```python
from build123d import *

# Parameters (mm, degrees)
SKETCH1_R               = 20
SKETCH1_R_2             = 14.25
SKETCH1_R_3             = 1.6
SKETCH1_W               = 2
SKETCH1_H               = 20
BOSS_EXTRUDE1_DEPTH     = 2
CUT_EXTRUDE3_DEPTH      = 171.89177862
CUT_EXTRUDE3_DEPTH_BACK = 171.89177862
SKETCH4_W               = 15
SKETCH4_H               = 2
CUT_EXTRUDE4_DEPTH      = 171.89177862
CUT_EXTRUDE4_DEPTH_BACK = 171.89177862
SKETCH5_R               = 14.25
SKETCH5_R_2             = 1.6


with BuildPart() as part:
    # Sketch1 → Boss-Extrude1 (new body)
    with BuildSketch(Plane.XY):
        Polygon((-158, -56), (-146.5, -56), (-146.5, -60), (-131.5, -60), (-131.5, -56), (-106.5, -56), (-106.5, -60), (-91.5, -60), (-91.5, -56), (-66.5, -56), (-66.5, -60), (-51.5, -60), (-51.5, -56), (-26.5, -56), (-26.5, -60), (-11.5, -60), (-11.5, -56), (11.5, -56), (11.5, -60), (26.5, -60), (26.5, -56), (51.5, -56), (51.5, -60), (66.5, -60), (66.5, -56), (91.5, -56), (91.5, -60), (106.5, -60), (106.5, -56), (131.5, -56), (131.5, -60), (146.5, -60), (146.5, -56), (158, -56), (158, -24), (160, -24), (160, -4), (158, -4), (158, 16), (160, 16), (160, 36), (158, 36), (158, 56), (146.5, 56), (146.5, 58), (131.5, 58), (131.5, 56), (106.5, 56), (106.5, 58), (91.5, 58), (91.5, 56), (66.5, 56), (66.5, 58), (51.5, 58), (51.5, 56), (26.5, 56), (26.5, 58), (11.5, 58), (11.5, 56), (-11.5, 56), (-11.5, 58), (-26.5, 58), (-26.5, 56), (-51.5, 56), (-51.5, 58), (-66.5, 58), (-66.5, 56), (-91.5, 56), (-91.5, 58), (-106.5, 58), (-106.5, 56), (-131.5, 56), (-131.5, 58), (-146.5, 58), (-146.5, 56), (-158, 56), (-158, 36), (-160, 36), (-160, 16), (-158, 16), (-158, -4), (-160, -4), (-160, -24), (-158, -24), align=None)
        with Locations((-120, -18)):
            Circle(SKETCH1_R, mode=Mode.SUBTRACT)
        with Locations((88, -31)):
            Circle(SKETCH1_R_2, mode=Mode.SUBTRACT)
        with Locations((73, -16)):
            Circle(SKETCH1_R_3, mode=Mode.SUBTRACT)
        with Locations((103, -16)):
            Circle(SKETCH1_R_3, mode=Mode.SUBTRACT)
        with Locations((73, -46)):
            Circle(SKETCH1_R_3, mode=Mode.SUBTRACT)
        with Locations((103, -46)):
            Circle(SKETCH1_R_3, mode=Mode.SUBTRACT)
        with Locations((-37, -14)):
            Rectangle(SKETCH1_W, SKETCH1_H, mode=Mode.SUBTRACT)
        with Locations((-37, 26)):
            Rectangle(SKETCH1_W, SKETCH1_H, mode=Mode.SUBTRACT)
    extrude(amount=BOSS_EXTRUDE1_DEPTH)

    # Sketch4 → Cut-Extrude3 (cut, two sides: drawn at the far end of the back side and taken through both)
    with BuildSketch(Plane.XY.offset(2).offset(-CUT_EXTRUDE3_DEPTH_BACK)):
        with Locations((-139, 57)):
            Rectangle(SKETCH4_W, SKETCH4_H)
        with Locations((-99, 57)):
            Rectangle(SKETCH4_W, SKETCH4_H)
        with Locations((-59, 57)):
            Rectangle(SKETCH4_W, SKETCH4_H)
        with Locations((-19, 57)):
            Rectangle(SKETCH4_W, SKETCH4_H)
        with Locations((19, 57)):
            Rectangle(SKETCH4_W, SKETCH4_H)
        with Locations((59, 57)):
            Rectangle(SKETCH4_W, SKETCH4_H)
        with Locations((99, 57)):
            Rectangle(SKETCH4_W, SKETCH4_H)
        with Locations((139, 57)):
            Rectangle(SKETCH4_W, SKETCH4_H)
    extrude(amount=CUT_EXTRUDE3_DEPTH + CUT_EXTRUDE3_DEPTH_BACK, mode=Mode.SUBTRACT)

    # Sketch5 → Cut-Extrude4 (cut, two sides: drawn at the far end of the back side and taken through both)
    with BuildSketch(Plane.XY.offset(2).offset(-CUT_EXTRUDE4_DEPTH_BACK)):
        with Locations((128, 26)):
            Circle(SKETCH5_R)
        with Locations((113, 41)):
            Circle(SKETCH5_R_2)
        with Locations((143, 41)):
            Circle(SKETCH5_R_2)
        with Locations((143, 11)):
            Circle(SKETCH5_R_2)
        with Locations((113, 11)):
            Circle(SKETCH5_R_2)
        with Locations((82, 26)):
            Circle(SKETCH5_R)
        with Locations((97, 11)):
            Circle(SKETCH5_R_2)
        with Locations((67, 11)):
            Circle(SKETCH5_R_2)
        with Locations((67, 41)):
            Circle(SKETCH5_R_2)
        with Locations((97, 41)):
            Circle(SKETCH5_R_2)
        with Locations((36, 26)):
            Circle(SKETCH5_R)
        with Locations((51, 11)):
            Circle(SKETCH5_R_2)
        with Locations((21, 11)):
            Circle(SKETCH5_R_2)
        with Locations((21, 41)):
            Circle(SKETCH5_R_2)
        with Locations((51, 41)):
            Circle(SKETCH5_R_2)
        with Locations((-10, 26)):
            Circle(SKETCH5_R)
        with Locations((5, 11)):
            Circle(SKETCH5_R_2)
        with Locations((-25, 11)):
            Circle(SKETCH5_R_2)
        with Locations((-25, 41)):
            Circle(SKETCH5_R_2)
        with Locations((5, 41)):
            Circle(SKETCH5_R_2)
    extrude(amount=CUT_EXTRUDE4_DEPTH + CUT_EXTRUDE4_DEPTH_BACK, mode=Mode.SUBTRACT)


solid = part.part
```
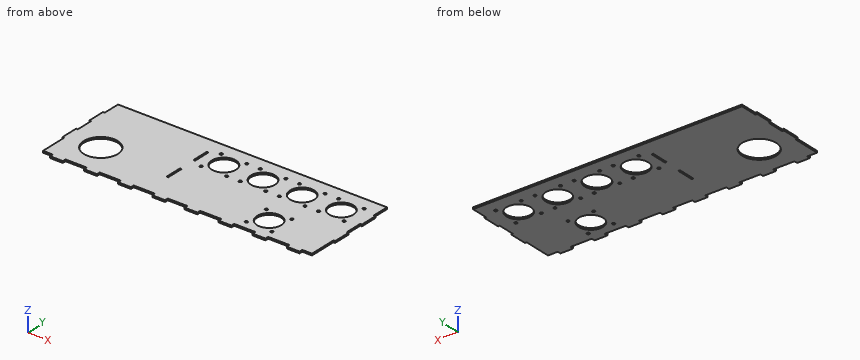
Work out the finished part from the listing and answer in its coordinate system (mm). Give positions to 0.01 mm unless a question says otherwise; leave off trailing zeros. Loops run counter-clockwise (first coordinate to the right, second up) from the corner with the lowest first, then second, coordinate; pieces in that order, holes last. Notation, with made-up numbers: M 60.25,87 L 112.25,87 A37 cw 112.25,125 Z; hole C 67,42.25 d1. An arc over 180 degrees is marked long. One line per item, written item: value. Start each with the question number.
1. Find section C-C (x = 82). Give the vertices of the cut face in (y, z).
2. Find section A-A (x = -120). Give the vertices of the cut face in (y, z).
3. Find section B-B (y = 26). Give the vertices of the cut face in (x, z).
4. Find section D-D (y = -21). Give the vertices of the cut face in (x, z).
5. Each of these flat-tipped pins is pushed along its axis until it touches: P1, Ø17, axis at x = 82, y = 26, coming from the -Z side; P2, Ø1, axis at x = 159.5, z = 1, coming from the +Y side; P3, Ø1, axis at x = 119.5, z = 1, coming from the -Y side; P4, Ø0.6, axis at x = 159, z = 1, coming from the -Y side. Where does it stop, or does it pass through?
6. Find the intervals of material crossed by probe 1 along Y at (x, z) = (-25, 1.15); probe 2 along Y at (x, z) = (103, 1.3); probe 3 along X at (y, z) = (26, 1.35), in increasing order.
Reported:
1. outline: M -56,0 L -43.93,0 L -43.93,2 L -56,2 Z; M -18.07,0 L 11.75,0 L 11.75,2 L -18.07,2 Z; M 40.25,0 L 56,0 L 56,2 L 40.25,2 Z
2. outline: M -56,0 L -38,0 L -38,2 L -56,2 Z; M 2,0 L 56,0 L 56,2 L 2,2 Z
3. outline: M -160,0 L -38,0 L -38,2 L -160,2 Z; M -36,0 L -24.25,0 L -24.25,2 L -36,2 Z; M 4.25,0 L 21.75,0 L 21.75,2 L 4.25,2 Z; M 50.25,0 L 67.75,0 L 67.75,2 L 50.25,2 Z; M 96.25,0 L 113.75,0 L 113.75,2 L 96.25,2 Z; M 142.25,0 L 160,0 L 160,2 L 142.25,2 Z
4. outline: M -160,0 L -139.77,0 L -139.77,2 L -160,2 Z; M -100.23,0 L -38,0 L -38,2 L -100.23,2 Z; M -36,0 L 77.85,0 L 77.85,2 L -36,2 Z; M 98.15,0 L 160,0 L 160,2 L 98.15,2 Z
5. P1: passes through
5. P2: stops at y = 36
5. P3: stops at y = -56
5. P4: stops at y = -24
6. probe 1: y = -60 to 9.4, 12.6 to 39.4, 42.6 to 56
6. probe 2: y = -60 to -47.6, -44.4 to -17.6, -14.4 to 56
6. probe 3: x = -160 to -38, -36 to -24.25, 4.25 to 21.75, 50.25 to 67.75, 96.25 to 113.75, 142.25 to 160
